Can you work these out from the model? Positions are in its coordinate system, mm. A direction names the side the tool comes from. Coordinates: 2 decimals unless noted, no trailing zeros. Write each loop counter-clockwise with the first axis right and the second up, starting at its lowest first coordinate (ties: lowest second). Pieces come first, ordered by that corner, then holes. Notation, with made-up numbers: (51, 11) -> (71, 11) arc R20 cw to (71, 29) -> close; hole circle Ø11 at (87.5, 14.5). An arc over 180 degrees is marked (long way). Use one line per item in the form item = value.
Autodesk Inventor part; units mm, degrees
ref_plane "YZ Plane" through (0, 0, 0) normal (1, 0, 0) x (0, 1, 0)
ref_plane "XZ Plane" through (0, 0, 0) normal (0, 1, 0) x (-1, 0, 0)
ref_plane "XY Plane" through (0, 0, 0) normal (0, 0, 1) x (1, 0, 0)
sketch "スケッチ1" plane through (0, 0, 0) normal (1, 0, 0) x (0, 1, 0)
  line L0 (50, 50) -> (-50, 50)
  line L1 (-50, 50) -> (-50, -50)
  line L2 (-50, -50) -> (50, -50)
  line L3 (50, -50) -> (50, 50)
  point P0 (0, 0)
  dimension "d0" = 100
  dimension "d2" = 100
  dimension "d3" = 50
  dimension "d4" = 50
extrude "押し出し1" add sketch "スケッチ1" along normal blind 11
sketch "スケッチ2" plane through (11, 0, 0) normal (1, 0, 0) x (0, 0, -1)
  line L0 (-50, 50) -> (-50, -50)
  line L1 (-50, -50) -> (50, -50)
  line L2 (50, -50) -> (50, 50)
  line L3 (50, 50) -> (-50, 50)
  line L4 (-25, -50) -> (-10, -35)
  line L5 (-10, -35) -> (15, -35)
  line L6 (15, -35) -> (50, -25.6218)
  line L7 (-50, 0) -> (-25, 0)
  line L8 (-25, 0) -> (-10, -15)
  line L9 (-10, -15) -> (12.367, -15)
  line L10 (12.367, -15) -> (30, -10.2752)
  line L11 (30, -10.2752) -> (30, 50)
  line L12 (-25, -50) -> (-50, -50)
  line L13 (-50, -50) -> (-50, 0)
  point P0 (0, 0)
  dimension "d7" = 135
  dimension "d8" = 135
  dimension "d9" = 25
  dimension "d10" = 25
  dimension "d11" = 50
  dimension "d16" = 165
  dimension "d17" = 20
  dimension "d18" = 20
  dimension "d89" = 20
  dimension "d90" = 25
extrude "押し出し2" cut sketch "スケッチ2" against normal blind 11 contours L7 L8 L9 L10 L11 L3 L2 L6 L5 L4 L1 L0 keep common part
sketch "スケッチ3" plane through (11, 0, 0) normal (1, 0, 0) x (0, 0, -1)
  line L0 (30, -10.2752) -> (30, 50)
  line L1 (12.367, -15) -> (30, -10.2752)
  line L2 (-10, -15) -> (12.367, -15)
  line L3 (-25, 0) -> (-10, -15)
  line L4 (-50, 0) -> (-25, 0)
  line L5 (-50, 0) -> (-50, -50)
  line L6 (-50, -50) -> (-25, -50)
  line L7 (-10, -35) -> (-25, -50)
  line L8 (15, -35) -> (-10, -35)
  line L9 (50, -25.6218) -> (15, -35)
  line L10 (50, -25.6218) -> (50, 50)
  line L11 (50, 50) -> (30, 50)
  circle A0 centre (-42.5, -7.5) radius 2
  circle A1 centre (-42.5, -42.5) radius 2
  circle A2 centre (-22.5, -12.5) radius 1.25
  circle A3 centre (-22.5, -37.5) radius 1.25
  arc A4 (36, 46) -> (44, 46) centre (40, 46) ccw
  line L12 (36, 46) -> (36, 50)
  line L13 (44, 46) -> (44, 50)
  point P0 (0, 0)
  dimension "d21" = 8
  dimension "d25" = 4
  dimension "d30" = 6
  dimension "d31" = 4
  dimension "d35" = 25
  dimension "d36" = 35
  dimension "d37" = 12.5
  dimension "d38" = 7.5
  dimension "d40" = 7.5
  dimension "d41" = 7.5
  dimension "d61" = 2.5
  dimension "d68" = 20
  dimension "d69" = 20
extrude "押し出し5" cut sketch "スケッチ3" against normal blind 11 contours L0 L11 L12 A4 L13 L10 L9 L8 L7 L6 L5 L4 L3 L2 L1 keep common part
sketch "スケッチ4" plane through (11, 0, 0) normal (1, 0, 0) x (0, 0, -1)
  line L0 (50, 50) -> (30, 50)
  circle A0 centre (33, 46) radius 1
  arc A1 (36, 46) -> (44, 46) centre (40, 46) ccw
  point P0 (0, 0)
  dimension "d47" = 4
  dimension "d49" = 2
  dimension "d64" = 7
hole "穴1" at (11, 46, -33) direction (-1, 0, 0) diameter 2 end through all
pattern_circular "円形状パターン2" count 5 over 180 about axis through (11, 46, -40) along (1, 0, 0) of "穴1"
sketch "スケッチ5" plane through (11, 0, 0) normal (1, 0, 0) x (0, 0, -1)
  line L0 (-10, -15) -> (12.367, -15)
  circle A0 centre (-22.5, -12.5) radius 1.25
  circle A1 centre (-22.5, -37.5) radius 1.25
  circle A2 centre (2.5, -20) radius 1.3
  circle A3 centre (2.5, -30) radius 1.3
  point P0 (0, 0)
  dimension "d70" = 2.6
  dimension "d74" = 5
  dimension "d75" = 10
  dimension "d91" = 25
  dimension "d92" = 25
hole "穴2" at (11, -20, -2.5) at (11, -30, -2.5) direction (-1, 0, 0) diameter 2.2 end through all
sketch "スケッチ6" plane through (11, 0, 0) normal (1, 0, 0) x (0, 0, -1)
  circle A0 centre (2.5, -20) radius 1.1
  circle A1 centre (2.5, -30) radius 1.1
  line L0 (12.367, -15) -> (30, -10.2752)
  line L1 (-10, -15) -> (12.367, -15)
  line L2 (-25, 0) -> (-10, -15)
  line L3 (-50, 0) -> (-25, 0)
  line L4 (-50, 0) -> (-50, -50)
  line L5 (-50, -50) -> (-25, -50)
  line L6 (-10, -35) -> (-25, -50)
  line L7 (15, -35) -> (-10, -35)
  line L8 (50, -25.6218) -> (15, -35)
  circle A2 centre (-22.5, -12.5) radius 1.25
  circle A3 centre (-22.5, -37.5) radius 1.25
  circle A4 centre (-42.5, -7.5) radius 2
  circle A5 centre (-42.5, -42.5) radius 2
  line L9 (0, -15) -> (0, -35)
  point P0 (0, 0)
  dimension "d93" = 10
extrude "押し出し6" cut sketch "スケッチ6" against normal blind 11 contours L1 L9 L7 L6 L5 L4 L3 L2 keep common part
sketch "スケッチ7" plane through (11, 0, 0) normal (1, 0, 0) x (0, 0, -1)
  line L0 (-10, -15) -> (0, -15)
  line L1 (-50, 0) -> (-50, -50)
  line L2 (-50, -50) -> (-25, -50)
  line L3 (-31, -12.5) -> (-31, -37.5)
  line L4 (-31, -37.5) -> (-18.0096, -30)
  line L5 (-31, -12.5) -> (-18.0096, -20)
  line L6 (-18.0096, -20) -> (-8.0096, -20)
  line L7 (-8.0096, -20) -> (-8.0096, -30)
  line L8 (-8.0096, -30) -> (-18.0096, -30)
  circle A0 centre (-42.5, -42.5) radius 2
  circle A1 centre (-42.5, -7.5) radius 2
  circle A2 centre (-22.5, -37.5) radius 1.25
  circle A3 centre (-22.5, -12.5) radius 1.25
  line L9 (0, -15) -> (0, -35)
  line L10 (-25, 0) -> (-10, -15)
  line L11 (-50, 0) -> (-25, 0)
  line L12 (-10, -35) -> (-25, -50)
  line L13 (0, -35) -> (-10, -35)
  point P0 (0, 0)
  dimension "d101" = 25
  dimension "d102" = 12.5
  dimension "d105" = 150
  dimension "d106" = 150
  dimension "d107" = 10
  dimension "d109" = 10
  dimension "d110" = 5
  dimension "d120" = 19
sketch "スケッチ8" plane through (11, 0, 0) normal (1, 0, 0) x (0, 0, -1)
  line L0 (0, -15) -> (0, -35)
  line L1 (-50, 0) -> (-25, 0)
  line L2 (0, -35) -> (-10, -35)
  line L3 (-36, -10.3812) -> (-36, -39.6188)
  line L4 (-36, -39.6188) -> (-44, -35)
  line L5 (-44, -35) -> (-44, -15)
  line L6 (-44, -15) -> (-36, -10.3812)
  point P0 (0, 0)
  dimension "d113" = 20
  dimension "d115" = 8
  dimension "d116" = 120
  dimension "d117" = 120
  dimension "d118" = 15
  dimension "d119" = 36
extrude "押し出し11" cut sketch "スケッチ7" against normal blind 11 keep common part
extrude "押し出し12" cut sketch "スケッチ8" against normal blind 11
fillet "フィレット1" radius 10 2 edges at (5.5, -20, 18.0096) (5.5, -30, 18.0096)
fillet "フィレット2" radius 2 8 edges at (5.5, -12.5, 31) (5.5, -37.5, 31) (5.5, -35, 44) (5.5, -15, 44) (5.5, -10.3812, 36) (5.5, -39.6188, 36) (5.5, -30, 8.0096) (5.5, -20, 8.0096)
properties part number "Arm_MiniLink_1" material "アセタール樹脂、白"
Q1. If I drill on line 1 (Z direction, x = 5.25, y = -22); line 2 (Y direction, x = 6.25, z = 22.5); line 3 (Y direction, x = 4.75, z = 42.5), over which ranges is the centre line in solid material (lowest first)? Write a range as from..to.
Return value:
line_1 = 0..8.01, 31..36, 44..50
line_2 = -47.5..-38.75, -36.25..-32.59, -17.41..-13.75, -11.25..-2.5
line_3 = -50..-44.5, -40.5..-35.87, -14.13..-9.5, -5.5..0
Q2. Suppose I cut it at D-D (y = -17). Write out the boundary of the cut face in (x, z).
Return value:
outline = (0, 0) -> (11, 0) -> (11, 23.21) -> (0, 23.21) -> close; (0, 31) -> (11, 31) -> (11, 36) -> (0, 36) -> close; (0, 44) -> (11, 44) -> (11, 50) -> (0, 50) -> close
Q3. Will these pins go through, and if not, where does the flat tip stop? pin 1 (2.5 mm diameter, centred on y = -7.5, z = 42.5, fed in from +X) (3 decimals); pin 2 (6 mm diameter, centred on x = 5, z = 13.5, fed in from -Y); pin 3 (1 mm diameter, centred on x = 5, y = -43, fed in from -Z); pin 4 (3 mm diameter, centred on x = 5.5, z = 6, fed in from -Y).
Return value:
pin_1 = through
pin_2 = -41.5
pin_3 = 17.5
pin_4 = -35
Q4. Suppose I cut it at B-B (x = 4.25). Give the number of separate pieces and of enclosed holes in the cut face, then the cut area to 3 significant figures.
Return value:
separate_pieces = 1
enclosed_holes = 6
area = 1,430 mm2
Q5. Suppose I cut it at A-A (z = 14.5). Write out the boundary of the cut face in (x, y), then the cut area to 3 significant figures.
Return value:
outline = (0, -39.5) -> (11, -39.5) -> (11, -30) -> (0, -30) -> close; (0, -20) -> (11, -20) -> (11, -10.5) -> (0, -10.5) -> close
area = 209 mm2
Q6. Thinking about a two-plate mould opening in Z: for faces 1 (the flat face through (5, -50, 38)), 2 (the cylindrical face through (5.42, -37.87, 36.97)), 3 (the flat face through (6, -7, 18)), which applies, released by +Z, released by -Z, zero draft, split by the parting line, or undercut?
Return value:
face_1 = zero draft
face_2 = undercut
face_3 = released by -Z
Q7. Suppose I cut it at C-C (y = -7.5). Write out the boundary of the cut face in (x, z), then the cut area to 4 significant figures.
Return value:
outline = (0, 17.5) -> (11, 17.5) -> (11, 40.5) -> (0, 40.5) -> close; (0, 44.5) -> (11, 44.5) -> (11, 50) -> (0, 50) -> close
area = 313.5 mm2
Q8. For faces 4 (the flat face through (6, 0, 38)), 5 (the flat face through (6, -15, 5)), 6 (the flat face through (6, -30, 13)), which set-ups out of +Z, -Z, +X, -X, +Y, -Y let a thin tool reach every point of the face, with its end or its side?
Return value:
face_4 = +Z, -Z, +X, -X, +Y
face_5 = -Z, +X, -X, +Y
face_6 = +X, -X
